CAD build for the part. Positions are in the model's coordinates, mm. Coordinates: 2 decimals unless noted, no trailing zeros. Loops run counter-clockwise (first coordinate to the right, second up) from the corner with the lowest first, then second, coordinate; pieces in that order, holes last. Notation, with made-up numbers: (63.5, 41) -> (116.5, 41) arc R28 cw to (116.5, 66) -> close; hole circle Ø6 at (71.5, 19). An arc over 180 degrees is marked (long way). Write each question's results on one line, items separated by ' | '.
```python
from build123d import *

# Parameters (mm, degrees)
SKETCH_1_R      = 2.9
SKETCH_1_R_2    = 0.4
EXTRUDE_1_DEPTH = 1


with BuildPart() as part:
    # Эскиз1 → Бобышка-Вытянуть1 (new body)
    with BuildSketch(Plane.XY):
        with BuildLine():
            Line((6.163674565, -12.692207796), (-2.163674565, -6.107792204))
            ThreePointArc((-2.163674565, -6.107792204), (-2.309633742, -6.027716241), (-2.473792357, -6))
            Line((-2.473792357, -6), (-64, -6))
            ThreePointArc((-64, -6), (-64.353553391, -5.853553391), (-64.5, -5.5))
            Line((-64.5, -5.5), (-64.5, 5.5))
            ThreePointArc((-64.5, 5.5), (-64.353553391, 5.853553391), (-64, 6))
            Line((-64, 6), (64, 6))
            ThreePointArc((64, 6), (64.353553391, 5.853553391), (64.5, 5.5))
            Line((64.5, 5.5), (64.5, -6))
            Line((64.5, -6), (64.5, -12.3))
            ThreePointArc((64.5, -12.3), (64.353553391, -12.653553391), (64, -12.8))
            Line((64, -12.8), (6.473792357, -12.8))
            ThreePointArc((6.473792357, -12.8), (6.309633742, -12.772283759), (6.163674565, -12.692207796))
        make_face()
        with Locations((-46, 0.2)):
            Circle(SKETCH_1_R, mode=Mode.SUBTRACT)
        with Locations((-52, 0.2)):
            Circle(SKETCH_1_R_2, mode=Mode.SUBTRACT)
    extrude(amount=EXTRUDE_1_DEPTH)


solid = part.part
```
Q1. Wall check: L1, parallel to Y at x = -46, z = 0.7; L2, parallel to X at y = -0.75, z = 0.6; L3, parallel to Y at x = -36, z = 0.8. Give the ranges that are in metal, low to high. Write a range as from..to.
Results are:
L1: -6..-2.7, 3.1..6 | L2: -64.5..-48.74, -43.26..64.5 | L3: -6..6
Q2. Pull direction X, two halves, no side cores. Call faces 1 (the cylindrical face through (-43.234, 1.071, 0.493)), 2 (the flat face through (2.058, -9.446, 0.493)), 3 (the flat face through (1, -1, 1)): +X half, -X half, draft (parallel to the pull), parting line (faces both ways), or undercut.
Results are:
face 1: undercut | face 2: -X half | face 3: draft
Q3. Cut at C-C on y = -10. Write the cut outline in (x, z).
Results are:
outline: (2.76, 0) -> (64.5, 0) -> (64.5, 1) -> (2.76, 1) -> close
Q4. Cut at A-A on x = -46. Write the cut outline in (y, z).
Results are:
outline: (-6, 0) -> (-2.7, 0) -> (-2.7, 1) -> (-6, 1) -> close; (3.1, 0) -> (6, 0) -> (6, 1) -> (3.1, 1) -> close
Q5. Cut at B-B on z = 0.4. Write the cut outline in (x, y), and give its area (3 significant figures).
Results are:
outline: (-64.5, -5.5) arc R0.5 ccw to (-64, -6) -> (-2.47, -6) arc R0.5 cw to (-2.16, -6.11) -> (6.16, -12.69) arc R0.5 ccw to (6.47, -12.8) -> (64, -12.8) arc R0.5 ccw to (64.5, -12.3) -> (64.5, 5.5) arc R0.5 ccw to (64, 6) -> (-64, 6) arc R0.5 ccw to (-64.5, 5.5) -> close; hole circle Ø0.8 at (-52, 0.2); hole circle Ø5.8 at (-46, 0.2) | area: 1,950 mm^2
